Geometry check sheet. Reference: the model listing, model coordinates, mm. Face numbers are marked on the shaded views. A direction names the side the tool comes from. Round coordinates to 2 decimals unless told otherwise and drop trailing zeros. Loops run counter-clockwise (first coordinate to the right, second up) from the corner with the lowest first, then second, coordinate; pieces in that order, holes last. Notation, with made-up numbers: (69, 60) -> (97, 60) arc R14 ccw to (97, 67) -> close; hole circle Ø7 at (10, 43.5). An arc over 180 degrees is marked (long way). Use one line per item in the form item = value.
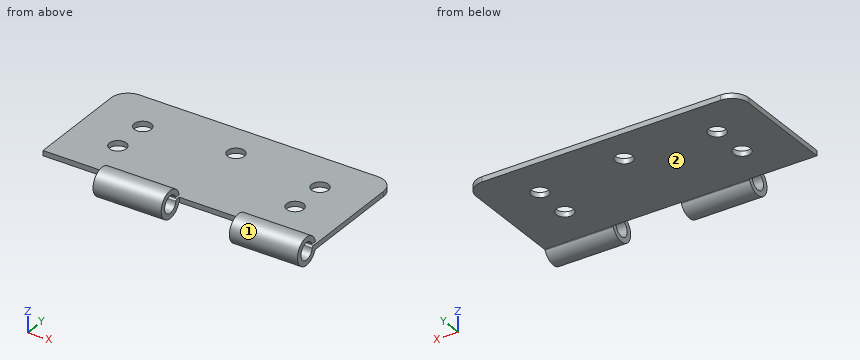
from build123d import *

# Parameters (mm, degrees)
BOSS_EXTRUDE1_DEPTH = 1.5
BOSS_EXTRUDE3_DEPTH = 20
LPATTERN1_COUNT     = 2
LPATTERN1_PITCH     = 40
SKETCH7_R           = 2.5
CUT_EXTRUDE1_DEPTH  = 48.610167833
SKETCH8_R           = 2.5
CUT_EXTRUDE2_DEPTH  = 48.610167833


with BuildPart() as part:
    # Sketch2 → Boss-Extrude1 (new body)
    with BuildSketch(Plane.XY):
        with BuildLine():
            Line((40, -17.5), (-40, -17.5))
            Line((-40, -17.5), (-40, 12.5))
            ThreePointArc((-40, 12.5), (-38.535533906, 16.035533906), (-35, 17.5))
            Line((-35, 17.5), (35, 17.5))
            ThreePointArc((35, 17.5), (38.535533906, 16.035533906), (40, 12.5))
            Line((40, 12.5), (40, -17.5))
        make_face()
    extrude(amount=BOSS_EXTRUDE1_DEPTH)

    # Sketch6 → Boss-Extrude3 (add)
    with BuildSketch(Plane(origin=(40, 0, 0), x_dir=(0, 0, -1), z_dir=(1, 0, 0))):
        with BuildLine():
            Line((-2.264835489, -17.585982761), (-2.264835489, -19.140334974))
            ThreePointArc((-2.264835489, -19.140334974), (-1.199434521, -23.988140772), (-1.072937624, -19.026256169))
            ThreePointArc((-1.072937624, -19.026256169), (-1.378463216, -18.858354721), (-1.5, -18.531604672))
            Line((-1.5, -18.531604672), (-1.5, -17.5))
            Line((-1.5, -17.5), (0, -17.5))
            Line((0, -17.5), (0, -17.598947109))
            ThreePointArc((0, -17.598947109), (0.041052608, -17.736209584), (0.150727898, -17.8283922))
            ThreePointArc((0.150727898, -17.8283922), (-1.837032289, -25.479523), (-2.264835489, -17.585982761))
        make_face()
    boss_extrude3 = extrude(amount=-BOSS_EXTRUDE3_DEPTH)

    # LPattern1: Boss-Extrude3 ×2
    with Locations(*[(-i * LPATTERN1_PITCH, 0, 0) for i in range(1, LPATTERN1_COUNT)]):
        add(boss_extrude3)

    # Sketch7 → Cut-Extrude1 (cut, through all)
    with BuildSketch(Plane.XY.offset(1.5)):
        with Locations((0, 7.5)):
            Circle(SKETCH7_R)
        with Locations((-26, -5.5)):
            Circle(SKETCH7_R)
        with Locations((26, -5.5)):
            Circle(SKETCH7_R)
    extrude(amount=-CUT_EXTRUDE1_DEPTH, mode=Mode.SUBTRACT)

    # Sketch8 → Cut-Extrude2 (cut, through all)
    with BuildSketch(Plane.XY.offset(1.5)):
        with Locations((-26, 5.5)):
            Circle(SKETCH8_R)
        with Locations((26, 5.5)):
            Circle(SKETCH8_R)
    extrude(amount=-CUT_EXTRUDE2_DEPTH, mode=Mode.SUBTRACT)


solid = part.part
1. Gauge pin test, flat ends, axial feed: pin 1 (4 mm diameter, centred on x = 30.5, y = 11, fed in from -Z); pin 2 (3 mm diameter, centred on x = 26, y = 5.5, fed in from -Z); pin 3 (8 mm diameter, centred on x = 5, y = -18, fed in from +Z); pin 4 (1.2 mm diameter, centred on x = -8.5, y = -18.5, fed in from -Z). Record the tip position at first contact, or that the pin passes through.
Return value:
pin_1 = 0
pin_2 = through
pin_3 = 1.5
pin_4 = -1.76
2. Tool access check on the marked faces 1 and 2. Record the directions out of +Z, -Z, +X, -X, +Y, -Y that give a thin tool (end or side, any length) a straight path to the whole face; none if there is none.
Return value:
face_1 = +X, -X
face_2 = -Z, +X, -X, +Y
3. Material ranges on line 1 along Y through (x, z) = (26, 0.7); line 2 along X through (y, z) = (-20.5, -1); line 3 along Z through (x, y) = (2, 14), recorded low to high.
Return value:
line_1 = -25.43 to -23.89, -19.11 to -8, -3 to 3, 8 to 17.5
line_2 = -20 to 0, 20 to 40
line_3 = 0 to 1.5
4. Section check A-A (y = -21.5). Record the boundary of the cut face in (x, z), then the cut area to 3 significant figures.
Return value:
outline = (-20, -2.56) -> (0, -2.56) -> (0, -1.06) -> (-20, -1.06) -> close; (-20, 3.94) -> (0, 3.94) -> (0, 5.44) -> (-20, 5.44) -> close; (20, -2.56) -> (40, -2.56) -> (40, -1.06) -> (20, -1.06) -> close; (20, 3.94) -> (40, 3.94) -> (40, 5.44) -> (20, 5.44) -> close
area = 120 mm2
5. Section check B-B (y = -5.5). Record the boundary of the cut face in (x, z).
Return value:
outline = (-40, 0) -> (-28.5, 0) -> (-28.5, 1.5) -> (-40, 1.5) -> close; (-23.5, 0) -> (23.5, 0) -> (23.5, 1.5) -> (-23.5, 1.5) -> close; (28.5, 0) -> (40, 0) -> (40, 1.5) -> (28.5, 1.5) -> close
6. Section check D-D (z = 3). Record the boundary of the cut face in (x, y).
Return value:
outline = (-20, -25.18) -> (0, -25.18) -> (0, -23.45) -> (-20, -23.45) -> close; (-20, -19.55) -> (0, -19.55) -> (0, -17.82) -> (-20, -17.82) -> close; (20, -25.18) -> (40, -25.18) -> (40, -23.45) -> (20, -23.45) -> close; (20, -19.55) -> (40, -19.55) -> (40, -17.82) -> (20, -17.82) -> close
7. Section check C-C (x = -26). Record the boundary of the cut face in (y, z).
Return value:
outline = (-17.5, 0) -> (-8, 0) -> (-8, 1.5) -> (-17.5, 1.5) -> close; (-3, 0) -> (3, 0) -> (3, 1.5) -> (-3, 1.5) -> close; (8, 0) -> (17.5, 0) -> (17.5, 1.5) -> (8, 1.5) -> close
